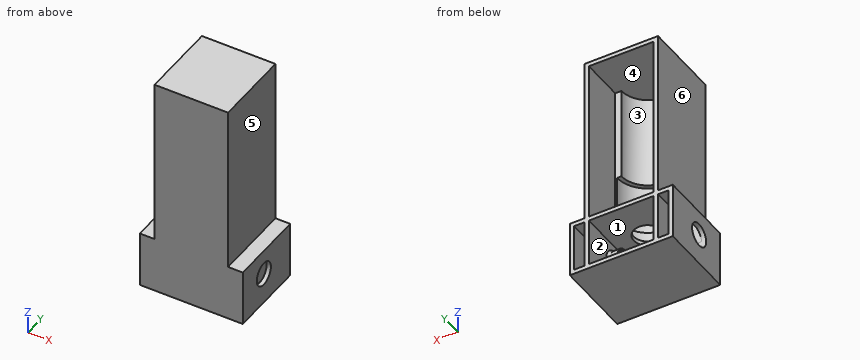
from build123d import *

# Parameters (mm, degrees)
BOSS_EXTRUDE1_START      = 15.24
BOSS_EXTRUDE1_DEPTH      = 38.1
SKETCH2_W                = 53.879496
SKETCH2_H                = 57.15
BOSS_EXTRUDE2_DEPTH      = 3.175
CUT_EXTRUDE2_DEPTH       = 68.189672735
CUT_EXTRUDE2_DEPTH_BACK  = 68.189672735
SKETCH3_R                = 8.5
SKETCH7_W                = 7.62
SKETCH7_H                = 9.935154996
BOSS_EXTRUDE7_DEPTH      = 1.5875
SKETCH8_W                = 53.879496
SKETCH8_H                = 57.15
BOSS_EXTRUDE8_DEPTH      = 127
CUT_EXTRUDE7_DEPTH       = 156.640901187
CUT_EXTRUDE7_DEPTH_BACK  = 156.640901187
SKETCH13_W               = 0.002356984
SKETCH13_H               = 126.769061331
CUT_EXTRUDE8_START       = -31.75
SKETCH14_W               = 47.527139016
SKETCH14_H               = 120.65
CUT_EXTRUDE8_DEPTH       = 31.75
CUT_EXTRUDE9_DEPTH       = 1.689066359
SKETCH18_W               = 13.97
SKETCH18_H               = 41.275
SKETCH18_W_2             = 7.62
SKETCH18_H_2             = 34.925
BOSS_EXTRUDE10_DEPTH     = 57.15
BOSS_EXTRUDE11_REACH     = 164.485
CUT_EXTRUDE11_DEPTH      = 166.168181283
CUT_EXTRUDE11_DEPTH_BACK = 166.168181283
SKETCH20_R               = 8.5


with BuildPart() as part:
    # Sketch1 → Boss-Extrude1 (new body)
    with BuildSketch(Plane.XY.offset(BOSS_EXTRUDE1_START)):
        Polygon((-26.939748, 0), (26.939748, 0), (26.939748, 6.35), (26.939748, 57.15), (23.764748, 57.15), (23.764748, 6.35), (-23.764748, 6.35), (-23.764748, 57.15), (-26.939748, 57.15), (-26.939748, 6.35), align=None)
    extrude(amount=-BOSS_EXTRUDE1_DEPTH)

    # Sketch2 → Boss-Extrude2 (add)
    with BuildSketch(Plane.XY.offset(-22.86)):
        with Locations((0, 28.575)):
            Rectangle(SKETCH2_W, SKETCH2_H)
    extrude(amount=BOSS_EXTRUDE2_DEPTH)

    # Sketch6 → Revolve2 (revolve)
    with BuildSketch(Plane.XY, mode=Mode.PRIVATE) as revolve2_sk:
        Polygon((-23.764748, 25.4), (-16.144748, 25.4), (-16.144748, 34.90000005), (-21.224748, 34.90000005), (-23.764748, 36.068), align=None)
        Polygon((23.764748, 36.068), (23.764748, 25.4), (16.144748, 25.4), (16.144748, 34.90000005), (21.224748, 34.90000005), align=None)
    revolve(revolve2_sk.sketch.rotate(Axis((-23.764748, 25.4, 0), (1, 0, 0)), 90), axis=Axis((-23.764748, 25.4, 0), (1, 0, 0)))

    # Sketch3 → Cut-Extrude2 (cut, two sides: drawn at the far end of the back side and taken through both)
    with BuildSketch(Plane(origin=(0, 0, 0), x_dir=(0, 0, -1), z_dir=(1, 0, 0)).offset(-CUT_EXTRUDE2_DEPTH_BACK)):
        with Locations((0, 25.4)):
            Circle(SKETCH3_R)
    extrude(amount=CUT_EXTRUDE2_DEPTH + CUT_EXTRUDE2_DEPTH_BACK, mode=Mode.SUBTRACT)

    # Sketch7 → Boss-Extrude7 (add, symmetric)
    with BuildSketch(Plane.XY):
        with Locations((-19.954748, 11.317577498)):
            Rectangle(SKETCH7_W, SKETCH7_H)
        with Locations((19.954748, 11.317577498)):
            Rectangle(SKETCH7_W, SKETCH7_H)
    extrude(amount=BOSS_EXTRUDE7_DEPTH, both=True)

    # Sketch8 → Boss-Extrude8 (add)
    with BuildSketch(Plane(origin=(0, 0, 15.24), x_dir=(-1, 0, 0), z_dir=(0, 0, -1))):
        with Locations((0, 28.575)):
            Rectangle(SKETCH8_W, SKETCH8_H)
    extrude(amount=-BOSS_EXTRUDE8_DEPTH)

    # Sketch9 → Cut-Revolve1 (revolve, cut)
    with BuildSketch(Plane(origin=(0, 0, 0), x_dir=(0, 0, -1), z_dir=(1, 0, 0))):
        Polygon((-70.6, 47.752), (-70.6, 44.577), (-139.065, 44.577), (-139.065, 25.4), (-70.104, 25.4), (0, 25.4), (0, 35.56), (-20.104066359, 35.56), (-20.104066359, 44.577), (-32.5, 44.577), (-32.5, 47.752), align=None)
    revolve(axis=Axis((0, 25.4, 0), (0, 0, 1)), mode=Mode.SUBTRACT)

    # Sketch13 → Cut-Extrude7 (cut, two sides: drawn at the far end of the back side and taken through both)
    with BuildSketch(Plane(origin=(0, 0, 0), x_dir=(-1, 0, 0), z_dir=(0, -1, 0)).offset(-CUT_EXTRUDE7_DEPTH_BACK)):
        with Locations((26.940926492, -78.855469335)):
            Rectangle(SKETCH13_W, SKETCH13_H)
        with Locations((-26.938569508, -78.855469335)):
            Rectangle(SKETCH13_W, SKETCH13_H)
    extrude(amount=CUT_EXTRUDE7_DEPTH + CUT_EXTRUDE7_DEPTH_BACK, mode=Mode.SUBTRACT)

    # Sketch14 → Cut-Extrude8 (cut)
    with BuildSketch(Plane(origin=(0, 57.15, 0), x_dir=(1, 0, 0), z_dir=(0, 1, 0)).offset(CUT_EXTRUDE8_START)):
        with Locations((-0.001178492, -78.74)):
            Rectangle(SKETCH14_W, SKETCH14_H)
    extrude(amount=CUT_EXTRUDE8_DEPTH, mode=Mode.SUBTRACT)

    # Sketch15 → Cut-Extrude9 (cut)
    with BuildSketch(Plane.XY.offset(20.104066359)):
        with BuildLine():
            Line((-10.16, 25.4), (-19.177, 25.4))
            ThreePointArc((-19.177, 25.4), (0, 6.223), (19.177, 25.4))
            Line((19.177, 25.4), (10.16, 25.4))
            ThreePointArc((10.16, 25.4), (0, 15.24), (-10.16, 25.4))
        make_face()
    extrude(amount=-CUT_EXTRUDE9_DEPTH, mode=Mode.SUBTRACT)

    # Sketch18 → Boss-Extrude10 (add)
    with BuildSketch(Plane(origin=(0, 0, 0), x_dir=(1, 0, 0), z_dir=(0, 1, 0))):
        with Locations((-30.749748, 2.2225)):
            Rectangle(SKETCH18_W, SKETCH18_H)
        with Locations((-30.749748, 2.2225)):
            Rectangle(SKETCH18_W_2, SKETCH18_H_2, mode=Mode.SUBTRACT)
    boss_extrude10 = extrude(amount=BOSS_EXTRUDE10_DEPTH)

    # Sketch19 → Boss-Extrude11 (add, up to next)
    with BuildSketch(Plane(origin=(-26.939748, 0, 0), x_dir=(0, 0, -1), z_dir=(1, 0, 0)), mode=Mode.PRIVATE) as boss_extrude11_sk1:
        with BuildLine():
            Line((1.5875, 17.049560266), (22.225, 20.972950206))
            Line((22.225, 20.972950206), (22.225, 0))
            Line((22.225, 0), (-15.24, 0))
            Line((-15.24, 0), (-15.24, 19.645033611))
            Line((-15.24, 19.645033611), (-1.5875, 17.049560266))
            ThreePointArc((-1.5875, 17.049560266), (0, 16.9), (1.5875, 17.049560266))
        make_face()
    boss_extrude11_tool1 = extrude(boss_extrude11_sk1.sketch, amount=-BOSS_EXTRUDE11_REACH, mode=Mode.PRIVATE) - part.part
    boss_extrude11 = boss_extrude11_tool1.solids().sort_by_distance((-26.939748, 9.331139, -3.822254))[0]
    add(boss_extrude11)

    # Mirror4: Boss-Extrude10, Boss-Extrude11 across plane
    add(boss_extrude10.mirror(Plane(origin=(0, 0, 0), x_dir=(0, 0, 1), z_dir=(1, 0, 0))))
    add(boss_extrude11.mirror(Plane(origin=(0, 0, 0), x_dir=(0, 0, 1), z_dir=(1, 0, 0))))

    # Sketch20 → Cut-Extrude11 (cut, two sides: drawn at the far end of the back side and taken through both)
    with BuildSketch(Plane(origin=(-23.764748, 0, 0), x_dir=(0, 0, -1), z_dir=(1, 0, 0)).offset(-CUT_EXTRUDE11_DEPTH_BACK)):
        with Locations((0, 25.4)):
            Circle(SKETCH20_R)
    extrude(amount=CUT_EXTRUDE11_DEPTH + CUT_EXTRUDE11_DEPTH_BACK, mode=Mode.SUBTRACT)


solid = part.part
Input: part model. Units: mm. Frame: model coordinates. Face numbers are marked on the shaded views. A direction names the side the tool comes from. Round coordinates to 2 decimals unless told otherwise and drop trailing zeros. Write each loop counter-clockwise with the first axis right and the second up, starting at its lowest first coordinate (ties: lowest second). Pieces come first, ordered by that corner, then holes.
1) Reachability of the marked faces 4, 5 and 6 from +Z, -Z, +X, -X, +Y, -Y: full face, straight path, thin tool, end or side. Return the list, or none.
2) Cut plane B-B (x = 0). Return the cut outline in (y, z) (3 decimals), then the cut area to 3 significant figures.
3) Cut plane D-D (y = 45). Return the cut outline in (x, z) (3 decimals), then the cut area to 3 significant figures.
4) Draft query along Y for the marked faces 1, 2 and 3. Return one class per face: pulls with the +Y half, pulls with the -Y half, needs draft (parallel to the pull), parting line crosses it, or undercut.
5) Cut plane A-A (z = 0). Count the separate pieces of the cut face and the enclosed holes in it, then the cut area to 3 significant figures.
6) Contact query for flat-ended pins moving along their axis: P1, Ø3, axis at y = 45, z = 112, coming from the +X side; P2, Ø5, axis at x = 20, z = 31.5, coming from the +Y side; P3, Ø9.5, axis at y = 41, z = 84, coming from the -X side. Output: stop coordinate, or through.
7) Ray query, L1, parallel to Z at x = -9, y = 41.5 (3 decimals); L2, parallel to X at y = 25.4, z = 16.95; L3, parallel to Z at x = 20, y = 25 (3 decimals). Return the intervals inside material, ascending.
8) Cut plane C-C (z = 121). Return the cut outline in (x, y), then the cut area to 3 significant figures.
Geometry says:
1. face 4: +Y
1. face 5: +Z, +X, +Y, -Y
1. face 6: +Z, -X, +Y, -Y
2. outline: (0, -22.86) - (57.15, -22.86) - (57.15, -19.685) - (6.35, -19.685) - (6.35, 15.24) - (15.24, 15.24) - (15.24, 18.415) - (6.223, 18.415) - (6.223, 32.5) - (3.048, 32.5) - (3.048, 70.6) - (6.223, 70.6) - (6.223, 139.065) - (57.15, 139.065) - (57.15, 142.24) - (0, 142.24) - close; (35.56, 15.24) - (57.15, 15.24) - (57.15, 18.415) - (35.56, 18.415) - close
2. area: 1,330 mm2
3. outline: (-37.735, -22.86) - (37.735, -22.86) - (37.735, 18.415) - (26.937, 18.415) - (26.937, 142.24) - (-26.94, 142.24) - (-26.94, 18.415) - (-37.735, 18.415) - close; hole (-34.56, -19.685) - (-26.94, -19.685) - (-26.94, 15.24) - (-34.56, 15.24) - close; hole (-23.765, -19.685) - (23.765, -19.685) - (23.765, 15.24) - (-23.765, 15.24) - close; hole (-23.765, 18.415) - (23.762, 18.415) - (23.762, 139.065) - (-23.765, 139.065) - close; hole (26.94, -19.685) - (34.56, -19.685) - (34.56, 15.24) - (26.94, 15.24) - close
3. area: 1,860 mm2
4. face 1: needs draft
4. face 2: undercut
4. face 3: pulls with the +Y half
5. separate pieces: 5
5. enclosed holes: 0
5. area: 1,250 mm2
6. P1: stops at x = 26.94
6. P2: stops at y = 25.4
6. P3: stops at x = -26.94
7. L1: z = -22.86 to -19.685, 15.24 to 18.415, 139.065 to 142.24
7. L2: x = -37.73 to -10.16, 10.16 to 37.73
7. L3: z = -22.86 to -19.685, -9.492 to -8.491, 8.491 to 9.492, 15.24 to 32.5, 70.6 to 142.24
8. outline: (-26.94, 0) - (26.94, 0) - (26.94, 57.15) - (23.76, 57.15) - (23.76, 25.4) - (19.18, 25.4) arc R19.18 cw to (-19.18, 25.4) - (-23.76, 25.4) - (-23.76, 57.15) - (-26.94, 57.15) - close
8. area: 992 mm2
